The model under review builds one solid part; all positions refer to its coordinate system, in mm. Face numbers are marked on the shaded views. A direction names the side the tool comes from. Coordinates: 2 decimals unless noted, no trailing zeros. Order: outer loops, then holes, each group sorted by start corner. A loop starts at its lowest first (then second) coordinate and runs counter-clockwise, first axis right, second up. Notation, with made-up numbers: (40, 68.25) -> (84, 68.25) arc R19 ccw to (84, 86.25) -> close; hole circle Ø7 at (71, -22). An arc over 180 degrees is marked (long way). Use one line per item in the form item = value. Start each with the question number.
(1) Take a section at A-A (y = 0). State the section outline as (x, z) points.
(2) Mouldability with a two-part tool opening along Y and no side actions: class the marked faces 3, 4 and 5 as +Y half, -Y half, draft (parallel to the pull), parting line (faces both ways), or undercut.
(3) For the marked faces 1 and 2, list the 3-axis set-ups (+Z, -Z, +X, -X, +Y, -Y) from which the entire face can be reached by the end or side of a thin tool; tool diameter is ignored.
(4) Wall thickness on line 1 along X through (y, z) = (-1, 2); line 2 along X through (y, z) = (1, -20); line 3 along Z through (x, y) = (0, 1.25): over which ranges is each line inside the solid? List them lowest first.
(5) Insertion check: pin 1 Ø5 at (x, z) = (-10.5, -15.5) entering from +Y; pin 2 Ø10 at (x, y) = (-19.5, -3) entering from +Z; pin 3 Ø11.5 at (x, z) = (0, -20) entering from -Y; pin 4 Ø1 at (y, z) = (18, 54) entering from -X. Each pin has a flat end and moves straight along its axis. Give the tip position at first contact, or say it passes through.
(6) Take a section at B-B (z = -20). State the section outline as (x, y) points.
(7) Take a section at D-D (y = -7.5). State the section outline as (x, z) points, then the cut area to 3 significant figures.
(8) Take a section at C-C (x = 0). State the section outline as (y, z) points.
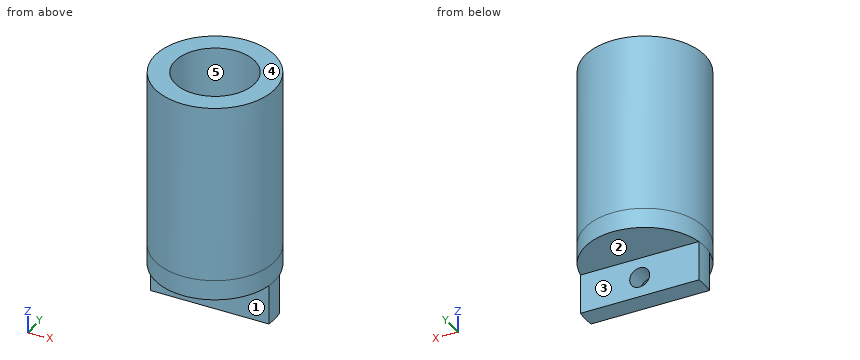
Autodesk Inventor part; units mm, degrees
ref_plane "YZ Plane" through (0, 0, 0) normal (1, 0, 0) x (0, 1, 0)
ref_plane "XZ Plane" through (0, 0, 0) normal (0, 1, 0) x (-1, 0, 0)
ref_plane "XY Plane" through (0, 0, 0) normal (0, 0, 1) x (1, 0, 0)
sketch "Эскиз1" plane through (0, 0, 0) normal (0, 0, 1) x (1, 0, 0)
  circle A0 centre (0, 0) radius 20
  circle A1 centre (0, 0) radius 30
  dimension "d0" = 40
  dimension "d1" = 10
extrude "Выдавливание1" add sketch "Эскиз1" along normal blind 90
sketch "Эскиз2" plane through (0, 0, 0) normal (0, 0, -1) x (-1, 0, 0)
  circle A0 centre (0, 0) radius 30
extrude "Выдавливание2" add sketch "Эскиз2" along normal blind 10
sketch "Эскиз3" plane through (0, 0, -10) normal (0, 0, -1) x (-1, 0, 0)
  circle A0 centre (0, 0) radius 30
  line L0 (-29.5804, 5) -> (29.5804, 5)
  line L1 (29.5804, -5) -> (-29.5804, -5)
  line L2 (42, 0) -> (-42, 0)
  dimension "d7" = 10
extrude "Выдавливание3" add sketch "Эскиз3" along normal blind 20 contours L2 A0 L0 | A0 L1 L2
sketch "Эскиз4" plane through (-29.5804, 5, -10) normal (0, 1, 0) x (1, 0, 0)
  line L0 (59.1608, 0) -> (0, 0)
  line L1 (59.1608, 0) -> (59.1608, 20)
  line L2 (0, 20) -> (59.1608, 20)
  line L3 (0, 0) -> (0, 20)
  line L4 (59.1608, 0) -> (59.1608, 20)
  line L5 (0, 0) -> (59.1608, 0)
  line L6 (0, 0) -> (0, 20)
  line L7 (0, 20) -> (59.1608, 20)
  circle A0 centre (29.5804, 10) radius 5
  point P0 (29.5804, -10)
  dimension "d11" = 10
extrude "Выдавливание4" cut sketch "Эскиз4" along normal through all both and the other way through all contours A0
properties part number "стакан_v2" material "Сталь"
Findings:
q1.outline = (-30, -30) -> (30, -30) -> (30, 90) -> (20, 90) -> (20, 0) -> (-20, 0) -> (-20, 90) -> (-30, 90) -> close; hole circle Ø10 at (0, -20)
q2.face_3 = +Y half
q2.face_4 = draft
q2.face_5 = undercut
q3.face_1 = -Z, +X, -X, -Y
q3.face_2 = -Z, +X, -X, +Y
q4.line_1 = -29.98 to -19.97, 19.97 to 29.98
q4.line_2 = -29.98 to -5, 5 to 29.98
q4.line_3 = -30 to -25, -15 to 0
q5.pin_1 = 5
q5.pin_2 = 90
q5.pin_3 = -5
q5.pin_4 = -24.37
q6.outline = (-29.58, -5) -> (-5, -5) -> (-5, 5) -> (-29.58, 5) arc R30 ccw to start; (5, -5) -> (29.58, -5) arc R30 ccw to (29.58, 5) -> (5, 5) -> close
q7.outline = (-29.05, -10) -> (29.05, -10) -> (29.05, 90) -> (18.54, 90) -> (18.54, 0) -> (-18.54, 0) -> (-18.54, 90) -> (-29.05, 90) -> close
q7.area = 2,470 mm²
q8.outline = (-30, -10) -> (-5, -10) -> (-5, -15) -> (5, -15) -> (5, -10) -> (30, -10) -> (30, 90) -> (20, 90) -> (20, 0) -> (-20, 0) -> (-20, 90) -> (-30, 90) -> close; (-5, -30) -> (5, -30) -> (5, -25) -> (-5, -25) -> close
